Geometry: final body of the model. Coordinates: model frame, mm. Coordinates: 2 decimals unless noted, no trailing zeros. Order: outer loops, then holes, each group sorted by start corner. A loop starts at its lowest first (then second) coordinate and runs counter-clockwise, first axis right, second up. Notation, with made-up numbers: (-19.75, 6) -> (27.25, 6) arc R27 cw to (27.25, 38) -> close; hole circle Ø6 at (65, 21.5). An arc over 180 degrees is marked (long way). Answer in a Markdown table with one row per item. Add a question column.
1) Contact query for flat-ended pins moving along their axis: P1, Ø5, axis at x = -5.5, y = 3, coming from the -Z side; P2, Ø1.5, axis at y = 1, z = 57.5, coming from the +X side. Output: stop coordinate, or through.
2) Section query B-B on y = -2.25. Return the cut outline in (x, z) (3 decimals).
3) Section query A-A on z = 29.5. Return the cut outline in (x, y) (3 decimals).
4) Ray query, line 1 (Y direction, x = 6.75, z = 8.5); line 2 (X direction, y = 3, z = 39.5); line 3 (Y direction, x = 5, z = 80.5). Return the intervals inside material, ascending. Write a range as from..to.
5) Section query C-C on y = 2. Return the cut outline in (x, z) (3 decimals), then the cut area to 3 significant figures.
```python
from build123d import *

# Parameters (mm, degrees)
F1_DEPTH = 85.725


with BuildPart() as f1:
    # F0 (on Top) → F1 (new body)
    with BuildSketch(Plane.XY):
        with BuildLine():
            ThreePointArc((5.4992612751, -3.1750000674), (6.1336289869, -1.643500974), (6.35, 0))
            ThreePointArc((6.35, 0), (6.1336289976, 1.6435009339), (5.4992613166, 3.1749999956))
            ThreePointArc((5.4992613166, 3.1749999956), (3.1750000022, 5.4992613128), (0, 6.35))
            ThreePointArc((0, 6.35), (-3.175000032, 5.4992612955), (-5.499261351, 3.174999936))
            ThreePointArc((-5.499261351, 3.174999936), (-6.35, 0), (-5.499261351, -3.174999936))
            ThreePointArc((-5.499261351, -3.174999936), (-3.175000032, -5.4992612955), (0, -6.35))
            ThreePointArc((0, -6.35), (3.1749999663, -5.4992613335), (5.4992612751, -3.1750000674))
        make_face()
        with BuildLine():
            ThreePointArc((5.4992613166, 3.1749999956), (6.1336289976, 1.6435009339), (6.35, 0))
            ThreePointArc((6.35, 0), (6.1336289869, -1.643500974), (5.4992612751, -3.1750000674))
            Line((5.4992612751, -3.1750000674), (7.3323484187, 0))
            Line((7.3323484187, 0), (5.4992613166, 3.1749999956))
        make_face()
        with BuildLine():
            ThreePointArc((0, 6.35), (3.1750000022, 5.4992613128), (5.4992613166, 3.1749999956))
            Line((5.4992613166, 3.1749999956), (3.6661742094, 6.35))
            Line((3.6661742094, 6.35), (0, 6.35))
        make_face()
        with BuildLine():
            Line((3.6661742094, -6.35), (5.4992612751, -3.1750000674))
            ThreePointArc((5.4992612751, -3.1750000674), (3.1749999663, -5.4992613335), (0, -6.35))
            Line((0, -6.35), (3.6661742094, -6.35))
        make_face()
        with BuildLine():
            ThreePointArc((-5.499261351, 3.174999936), (-3.175000032, 5.4992612955), (0, 6.35))
            Line((0, 6.35), (-3.6661742094, 6.35))
            Line((-3.6661742094, 6.35), (-5.499261351, 3.174999936))
        make_face()
        with BuildLine():
            Line((-3.6661742094, -6.35), (0, -6.35))
            ThreePointArc((0, -6.35), (-3.175000032, -5.4992612955), (-5.499261351, -3.174999936))
            Line((-5.499261351, -3.174999936), (-3.6661742094, -6.35))
        make_face()
        with BuildLine():
            ThreePointArc((-5.499261351, -3.174999936), (-6.35, 0), (-5.499261351, 3.174999936))
            Line((-5.499261351, 3.174999936), (-7.3323484187, 0))
            Line((-7.3323484187, 0), (-5.499261351, -3.174999936))
        make_face()
    extrude(amount=F1_DEPTH)


solid = f1.part
```
Result:
| question | item | result |
|---|---|---|
| 1 | P1 | z = 0 |
| 1 | P2 | x = 7.19 |
| 2 | outline | (-6.033, 0) -> (6.033, 0) -> (6.033, 85.725) -> (-6.033, 85.725) -> close |
| 3 | outline | (-7.332, 0) -> (-3.666, -6.35) -> (3.666, -6.35) -> (7.332, 0) -> (3.666, 6.35) -> (-3.666, 6.35) -> close |
| 4 | line 1 | -1.01..1.01 |
| 4 | line 2 | -5.6..5.6 |
| 4 | line 3 | -4.04..4.04 |
| 5 | outline | (-6.178, 0) -> (6.178, 0) -> (6.178, 85.725) -> (-6.178, 85.725) -> close |
| 5 | area | 1,060 mm2 |
